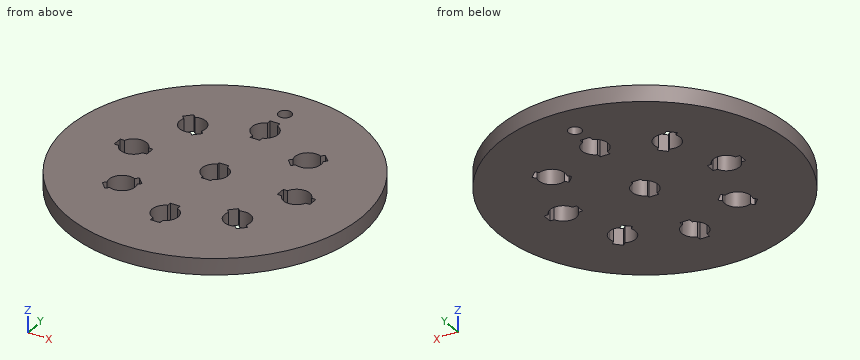
from build123d import *

# Parameters (mm, degrees)
F0_R     = 45
F0_R_2   = 2
F1_DEPTH = 2.5


with BuildPart() as f1:
    # F0 (on Top) → F1 (new body, symmetric)
    with BuildSketch(Plane.XY):
        Circle(F0_R)
        with BuildLine():
            Line((-15.202796, -13.081475), (-13.081475, -15.202796))
            Line((-13.081475, -15.202796), (-13.994987, -16.116308))
            ThreePointArc((-13.994987, -16.116308), (-13.757802, -16.881029), (-13.67767, -17.67767))
            ThreePointArc((-13.67767, -17.67767), (-15.469214, -21.012744), (-19.239031, -21.360352))
            Line((-19.239031, -21.360352), (-20.152543, -22.273864))
            Line((-20.152543, -22.273864), (-22.273864, -20.152543))
            Line((-22.273864, -20.152543), (-21.360352, -19.239031))
            ThreePointArc((-21.360352, -19.239031), (-20.506097, -14.849242), (-16.116308, -13.994987))
            Line((-16.116308, -13.994987), (-15.202796, -13.081475))
        make_face(mode=Mode.SUBTRACT)
        with BuildLine():
            ThreePointArc((1.5, -21.291901), (3.316625, -22.763932), (4, -25))
            ThreePointArc((4, -25), (3.316625, -27.236068), (1.5, -28.708099))
            Line((1.5, -28.708099), (1.5, -30))
            Line((1.5, -30), (-1.5, -30))
            Line((-1.5, -30), (-1.5, -28.708099))
            ThreePointArc((-1.5, -28.708099), (-4, -25), (-1.5, -21.291901))
            Line((-1.5, -21.291901), (-1.5, -20))
            Line((-1.5, -20), (1.5, -20))
            Line((1.5, -20), (1.5, -21.291901))
        make_face(mode=Mode.SUBTRACT)
        with BuildLine():
            Line((13.081475, -15.202796), (15.202796, -13.081475))
            Line((15.202796, -13.081475), (16.116308, -13.994987))
            ThreePointArc((16.116308, -13.994987), (19.886125, -14.342595), (21.67767, -17.67767))
            ThreePointArc((21.67767, -17.67767), (21.597537, -18.47431), (21.360352, -19.239031))
            Line((21.360352, -19.239031), (22.273864, -20.152543))
            Line((22.273864, -20.152543), (20.152543, -22.273864))
            Line((20.152543, -22.273864), (19.239031, -21.360352))
            ThreePointArc((19.239031, -21.360352), (14.849242, -20.506097), (13.994987, -16.116308))
            Line((13.994987, -16.116308), (13.081475, -15.202796))
        make_face(mode=Mode.SUBTRACT)
        with BuildLine():
            Line((-20, 1.5), (-20, -1.5))
            Line((-20, -1.5), (-21.291901, -1.5))
            ThreePointArc((-21.291901, -1.5), (-25, -4), (-28.708099, -1.5))
            Line((-28.708099, -1.5), (-30, -1.5))
            Line((-30, -1.5), (-30, 1.5))
            Line((-30, 1.5), (-28.708099, 1.5))
            ThreePointArc((-28.708099, 1.5), (-25, 4), (-21.291901, 1.5))
            Line((-21.291901, 1.5), (-20, 1.5))
        make_face(mode=Mode.SUBTRACT)
        with BuildLine():
            Line((-13.081475, 15.202796), (-15.202796, 13.081475))
            Line((-15.202796, 13.081475), (-16.116308, 13.994987))
            ThreePointArc((-16.116308, 13.994987), (-20.506097, 14.849242), (-21.360352, 19.239031))
            Line((-21.360352, 19.239031), (-22.273864, 20.152543))
            Line((-22.273864, 20.152543), (-20.152543, 22.273864))
            Line((-20.152543, 22.273864), (-19.239031, 21.360352))
            ThreePointArc((-19.239031, 21.360352), (-15.469214, 21.012744), (-13.67767, 17.67767))
            ThreePointArc((-13.67767, 17.67767), (-13.757802, 16.881029), (-13.994987, 16.116308))
            Line((-13.994987, 16.116308), (-13.081475, 15.202796))
        make_face(mode=Mode.SUBTRACT)
        with BuildLine():
            ThreePointArc((1.5, 3.708099), (3.316625, 2.236068), (4, 0))
            ThreePointArc((4, 0), (3.316625, -2.236068), (1.5, -3.708099))
            Line((1.5, -3.708099), (1.5, -4.5))
            Line((1.5, -4.5), (-1.5, -4.5))
            Line((-1.5, -4.5), (-1.5, -3.708099))
            ThreePointArc((-1.5, -3.708099), (-4, 0), (-1.5, 3.708099))
            Line((-1.5, 3.708099), (-1.5, 4.5))
            Line((-1.5, 4.5), (1.5, 4.5))
            Line((1.5, 4.5), (1.5, 3.708099))
        make_face(mode=Mode.SUBTRACT)
        with BuildLine():
            Line((15.202796, 13.081475), (13.081475, 15.202796))
            Line((13.081475, 15.202796), (13.994987, 16.116308))
            ThreePointArc((13.994987, 16.116308), (14.849242, 20.506097), (19.239031, 21.360352))
            Line((19.239031, 21.360352), (20.152543, 22.273864))
            Line((20.152543, 22.273864), (22.273864, 20.152543))
            Line((22.273864, 20.152543), (21.360352, 19.239031))
            ThreePointArc((21.360352, 19.239031), (21.597537, 18.47431), (21.67767, 17.67767))
            ThreePointArc((21.67767, 17.67767), (19.886125, 14.342595), (16.116308, 13.994987))
            Line((16.116308, 13.994987), (15.202796, 13.081475))
        make_face(mode=Mode.SUBTRACT)
        with BuildLine():
            Line((20, -1.5), (20, 1.5))
            Line((20, 1.5), (21.291901, 1.5))
            ThreePointArc((21.291901, 1.5), (25, 4), (28.708099, 1.5))
            Line((28.708099, 1.5), (30, 1.5))
            Line((30, 1.5), (30, -1.5))
            Line((30, -1.5), (28.708099, -1.5))
            ThreePointArc((28.708099, -1.5), (25, -4), (21.291901, -1.5))
            Line((21.291901, -1.5), (20, -1.5))
        make_face(mode=Mode.SUBTRACT)
        with BuildLine():
            Line((1.5, 20), (-1.5, 20))
            Line((-1.5, 20), (-1.5, 21.291901))
            ThreePointArc((-1.5, 21.291901), (-4, 25), (-1.5, 28.708099))
            Line((-1.5, 28.708099), (-1.5, 30))
            Line((-1.5, 30), (1.5, 30))
            Line((1.5, 30), (1.5, 28.708099))
            ThreePointArc((1.5, 28.708099), (3.316625, 27.236068), (4, 25))
            ThreePointArc((4, 25), (3.316625, 22.763932), (1.5, 21.291901))
            Line((1.5, 21.291901), (1.5, 20))
        make_face(mode=Mode.SUBTRACT)
        with Locations((0, 35)):
            Circle(F0_R_2, mode=Mode.SUBTRACT)
    extrude(amount=F1_DEPTH, both=True)


solid = f1.part
The model under review builds one solid part; all positions refer to its coordinate system, in mm. Round coordinates to 2 decimals unless told otherwise and drop trailing zeros. Order: outer loops, then holes, each group sorted by start corner. A loop starts at its lowest first (then second) coordinate and runs counter-clockwise, first axis right, second up. Notation, with made-up numbers: (80.5, -10.5) -> (96.5, -10.5) arc R37 cw to (96.5, 25.5) -> close; hole circle Ø4 at (-7, 72.5). An arc over 180 degrees is marked (long way). Write item = value, one per line. Start each with the question number.
Item 1: Consider section B-B on y = 35. Write out the cut boundary in (x, z).
Item 2: Consider section C-C on x = 27. Write out the cut boundary in (y, z).
Item 3: Consider section D-D on z = 0.75. Count the separate pieces of the cut face and the enclosed holes in it, plus the area to 3 significant figures.
Item 4: For line 1 along Y through (x, z) = (0, 0.2); line 2 along X through (y, z) = (17.5, -1.3); line 3 along X through (y, z) = (13.5, -0.25), list the stretches that pass through material, from the lowest coordinate up.
Item 5: Clearance check with flat-ended pins moving along their axes: pin 1 Ø0.6 at (x, z) = (-29.5, -0.5) entering from -Y; pin 2 Ø3 at (x, y) = (0, 35) entering from +Z; pin 3 Ø0.6 at (x, z) = (-21, 0.5) entering from +Y; pin 4 Ø1.5 at (x, z) = (0, 1) entering from +Y. State where each tip first meets the part, or that it passes through.
Item 6: Consider section A-A on x = 0. Write out the cut boundary in (y, z), plus the area to 3 significant figures.
Conclusion:
q1.outline = (-28.28, -2.5) -> (-2, -2.5) -> (-2, 2.5) -> (-28.28, 2.5) -> close; (2, -2.5) -> (28.28, -2.5) -> (28.28, 2.5) -> (2, 2.5) -> close
q2.outline = (-36, -2.5) -> (-3.46, -2.5) -> (-3.46, 2.5) -> (-36, 2.5) -> close; (3.46, -2.5) -> (36, -2.5) -> (36, 2.5) -> (3.46, 2.5) -> close
q3.separate_pieces = 1
q3.enclosed_holes = 10
q3.area = 5,840 mm2
q4.line_1 = -45 to -30, -20 to -4.5, 4.5 to 20, 30 to 33, 37 to 45
q4.line_2 = -41.46 to -21.67, -13.68 to 13.68, 21.67 to 41.46
q4.line_3 = -42.93 to -15.62, -14.78 to 14.78, 15.62 to 42.93
q5.pin_1 = -34.24
q5.pin_2 = through
q5.pin_3 = 39.96
q5.pin_4 = 45
q6.outline = (-45, -2.5) -> (-30, -2.5) -> (-30, 2.5) -> (-45, 2.5) -> close; (-20, -2.5) -> (-4.5, -2.5) -> (-4.5, 2.5) -> (-20, 2.5) -> close; (4.5, -2.5) -> (20, -2.5) -> (20, 2.5) -> (4.5, 2.5) -> close; (30, -2.5) -> (33, -2.5) -> (33, 2.5) -> (30, 2.5) -> close; (37, -2.5) -> (45, -2.5) -> (45, 2.5) -> (37, 2.5) -> close
q6.area = 285 mm2
